Verification items for this drawing (mm, ordinates from the low corner). A direction names the side the tool comes from. Give positions to 0.01 mm unless a question says otherwise; leave off trailing zeros. Loops run counter-clockwise (first coordinate to the right, second up) from the corner with the lowest first, then second, coordinate; pieces in that order, holes last. Notation, with made-up numbers: M 56.5,46 L 69.5,46 A9 cw 69.5,53 Z; hole C 20,57 d4. An arc over 180 degrees is marked long. Write each question's results on one line, items separated by ' | '. Start each with the question number.
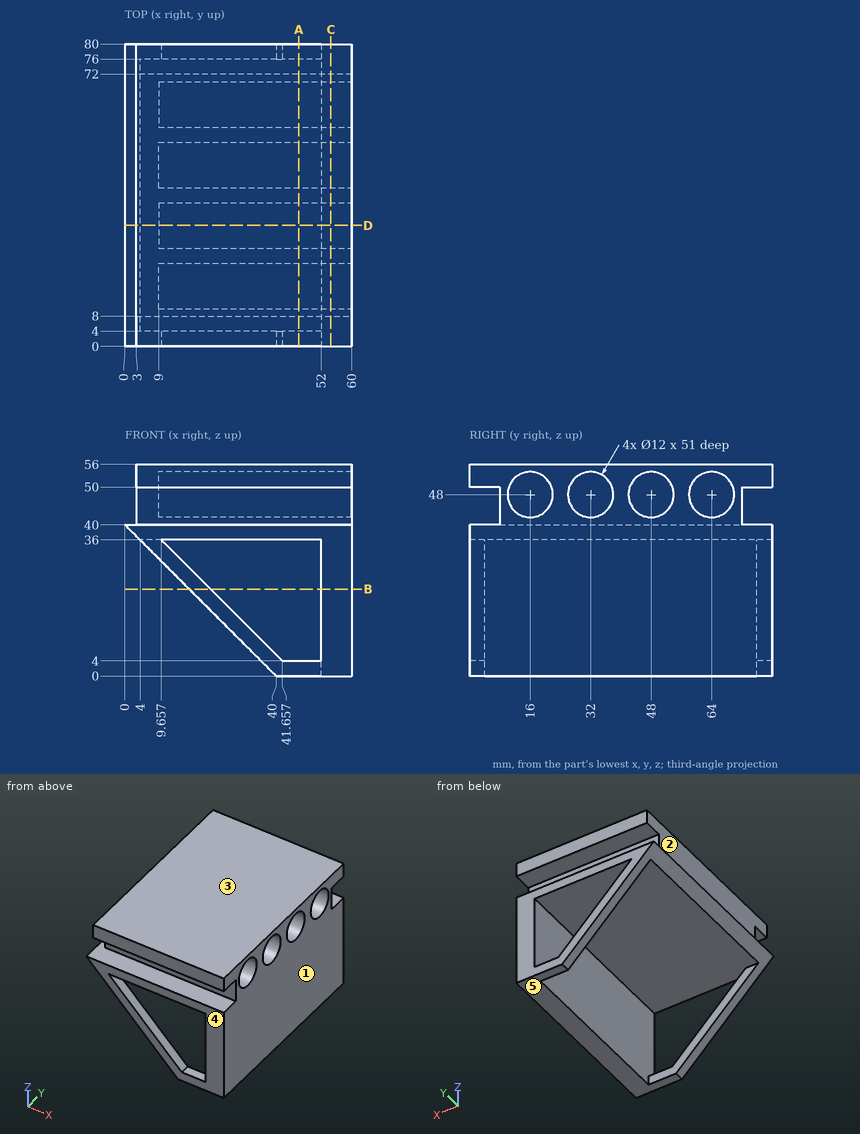
1. Section check B-B, the plane z = 23. Record the boundary of the cut face in (x, y), plus the area to 3 significant figures.
2. Section check A-A, the plane x = 46. Record the boundary of the cut face in (y, z), plus the area to 3 significant figures.
3. Section check D-D, the plane y = 32. Record the boundary of the cut face in (x, z), plus the area to 3 significant figures.
4. Section check C-C, the plane x = 54.5. Record the boundary of the cut face in (y, z).
5. Set-up check for the marked faces 1 and 2: record each of +Z, -Z, +X, -X, +Y, -Y from which the full face is reachable in a straight line by a thin tool's end or side.
6. Thickness scan on probe 1 along Y at (x, z) = (24.5, 48); probe 2 along Z at (x, y) = (43.5, 77.5); probe 3 along Y at (x, z) = (57.5, 42.5). Record the ranges inside material, lowest first.
7. Depth check by flat-ended pin: pin 1 Ø5 at (x, z) = (18, 43) entering from +Y; pin 2 Ø5 at (x, z) = (37.5, 47) entering from -Y; pin 3 Ø17.5 at (y, z) = (54, 46) entering from -X. Enter the tip coordinate at first touch or a pass-through.
8. Release check for a two-part mould opening along Z. For the marked faces 3, 4 and 5 record: released by +Z, released by -Z, zero draft, split by the parting line, or undercut.
Filled sheet:
1) outline: M 17,0 L 22.66,0 L 22.66,4 L 17,4 Z; M 17,76 L 22.66,76 L 22.66,80 L 17,80 Z; M 52,0 L 60,0 L 60,80 L 52,80 Z | area: 685 mm2
2) outline: M 0,0 L 4,0 L 4,4 L 0,4 Z; M 0,36 L 80,36 L 80,40 L 72,40 L 72,50 L 80,50 L 80,56 L 0,56 L 0,50 L 8,50 L 8,40 L 0,40 Z; M 76,0 L 80,0 L 80,4 L 76,4 Z; hole C 16,48 d12; hole C 32,48 d12; hole C 48,48 d12; hole C 64,48 d12 | area: 1,020 mm2
3) outline: M 0,40 L 4,36 L 52,36 L 52,0 L 60,0 L 60,42 L 9,42 L 9,54 L 60,54 L 60,56 L 3,56 L 3,40 Z | area: 820 mm2
4) outline: M 0,0 L 80,0 L 80,40 L 72,40 L 72,50 L 80,50 L 80,56 L 0,56 L 0,50 L 8,50 L 8,40 L 0,40 Z; hole C 16,48 d12; hole C 32,48 d12; hole C 48,48 d12; hole C 64,48 d12
5) face 1: +Z, -Z, +X, +Y, -Y | face 2: +Z, -X, +Y, -Y
6) probe 1: 8 to 10, 22 to 26, 38 to 42, 54 to 58, 70 to 72 | probe 2: 0 to 4, 36 to 40, 50 to 56 | probe 3: 8 to 13.6, 18.4 to 29.6, 34.4 to 45.6, 50.4 to 61.6, 66.4 to 72
7) pin 1: y = 72 | pin 2: y = 8 | pin 3: x = 0
8) face 3: released by +Z | face 4: zero draft | face 5: released by -Z
